```python
from build123d import *

# Parameters (mm, degrees)
SKETCH1_R                = 1.75
BOSS_EXTRUDE1_DEPTH      = 1.5
BOSS_EXTRUDE2_DEPTH      = 72
BOSS_EXTRUDE3_DEPTH      = 1.5
BOSS_EXTRUDE3_DEPTH_BACK = 1.5
BOSS_EXTRUDE4_DEPTH      = 2
SKETCH5_R                = 1.75
CUT_EXTRUDE1_DEPTH       = 2
CUT_EXTRUDE2_DEPTH       = 148.332054879
CUT_EXTRUDE2_DEPTH_BACK  = 148.332054879
SKETCH6_W                = 72
SKETCH6_H                = 11.553195909
BOSS_EXTRUDE6_START      = -2
SKETCH7_W                = 3
SKETCH7_H                = 4
BOSS_EXTRUDE6_DEPTH      = 2.5
FILLET1_R                = 2
CHAMFER1_SIZE            = 1
FILLET2_R                = 8
SKETCH8_W                = 35
SKETCH8_H                = 19.946804091
CUT_EXTRUDE3_DEPTH       = 22.4262221


with BuildPart() as part:
    # Sketch1 → Boss-Extrude1 (new body)
    with BuildSketch(Plane.XY):
        with BuildLine():
            Line((-31.5, -134.5), (31.5, -134.5))
            Line((31.5, -134.5), (36, -134.5))
            Line((36, -134.5), (36, -132.049019419))
            ThreePointArc((36, -132.049019419), (37.374296294, -129.5), (36, -126.950980581))
            Line((36, -126.950980581), (36, -6.049019419))
            ThreePointArc((36, -6.049019419), (37.33874188, -3.5), (36, -0.950980581))
            Line((36, -0.950980581), (36, 0))
            Line((36, 0), (-36, 0))
            Line((-36, 0), (-36, -0.950980581))
            ThreePointArc((-36, -0.950980581), (-37.339851511, -3.504206195), (-35.994020506, -6.054285021))
            Line((-35.994020506, -6.054285021), (-36, -126.950980581))
            ThreePointArc((-36, -126.950980581), (-37.376731289, -129.5), (-36, -132.049019419))
            Line((-36, -132.049019419), (-36, -134.5))
            Line((-36, -134.5), (-31.5, -134.5))
        make_face()
        with Locations((-34.328609587, -129.5)):
            Circle(SKETCH1_R, mode=Mode.SUBTRACT)
        with Locations((34.323211043, -129.5)):
            Circle(SKETCH1_R, mode=Mode.SUBTRACT)
        with Locations((34.242652207, -3.5)):
            Circle(SKETCH1_R, mode=Mode.SUBTRACT)
        with Locations((-34.244120111, -3.500578956)):
            Circle(SKETCH1_R, mode=Mode.SUBTRACT)
    extrude(amount=BOSS_EXTRUDE1_DEPTH)

    # Sketch2 → Boss-Extrude2 (add)
    with BuildSketch(Plane.ZY.offset(36)):
        Polygon((1.5, -134.5), (1.5, -136.7), (-40, -136.7), (-40, -134.7), (0, -134.7), (0, -134.5), (0, -132.049019419), (1.5, -132.049019419), align=None)
    extrude(amount=-BOSS_EXTRUDE2_DEPTH)

    # Sketch3 → Boss-Extrude3 (add, two sides: drawn at the far end of the back side and taken through both)
    with BuildSketch(Plane(origin=(0, 0, 0), x_dir=(0, 0, -1), z_dir=(1, 0, 0)).offset(-BOSS_EXTRUDE3_DEPTH_BACK)):
        Polygon((0, -119.7), (15, -134.7), (0, -134.7), align=None)
    extrude(amount=BOSS_EXTRUDE3_DEPTH + BOSS_EXTRUDE3_DEPTH_BACK)

    # Sketch4 → Boss-Extrude4 (add)
    with BuildSketch(Plane.XZ.offset(136.7)):
        with BuildLine():
            Line((-36, -17.152805247), (-36, -22.963011674))
            ThreePointArc((-36, -22.963011674), (-37.650416645, -20.05790846), (-36, -17.152805247))
        make_face()
        with BuildLine():
            Line((36, -17.152805247), (36, -22.963011674))
            ThreePointArc((36, -22.963011674), (37.68082264, -20.05790846), (36, -17.152805247))
        make_face()
    extrude(amount=-BOSS_EXTRUDE4_DEPTH)

    # Sketch5 → Cut-Extrude1 (cut)
    with BuildSketch(Plane.XZ.offset(136.7)):
        with Locations(Location((-34.253947115, -19.946804091, 0), (0, 0, 270))):
            Circle(SKETCH5_R)
        with Locations(Location((34.288977705, -19.889159472, 0), (0, 0, 270))):
            Circle(SKETCH5_R)
    extrude(amount=-CUT_EXTRUDE1_DEPTH, mode=Mode.SUBTRACT)

    # Sketch6 → Cut-Extrude2 (cut, two sides: drawn at the far end of the back side and taken through both)
    with BuildSketch(Plane.XZ.offset(136.7).offset(-CUT_EXTRUDE2_DEPTH_BACK)):
        with Locations((0, -34.223402046)):
            Rectangle(SKETCH6_W, SKETCH6_H)
    extrude(amount=CUT_EXTRUDE2_DEPTH + CUT_EXTRUDE2_DEPTH_BACK, mode=Mode.SUBTRACT)

    # Sketch7 → Boss-Extrude6 (add)
    with BuildSketch(Plane.XZ.offset(136.7).offset(BOSS_EXTRUDE6_START)):
        with Locations((-29.8, -26.446804091)):
            Rectangle(SKETCH7_W, SKETCH7_H)
        with Locations((29.8, -26.446804091)):
            Rectangle(SKETCH7_W, SKETCH7_H)
    extrude(amount=-BOSS_EXTRUDE6_DEPTH)

    # Fillet1
    fillet1_edges = [part.edges().sort_by_distance(p)[0] for p in [
        (36, -135.7, -28.446804091),
        (-36, -135.7, -28.446804091),
    ]]
    fillet(fillet1_edges, radius=FILLET1_R)

    # Chamfer1
    chamfer1_edges = [part.edges().sort_by_distance(p)[0] for p in [
        (-29.8, -134.7, -24.446804091),
        (-29.8, -132.2, -24.446804091),
        (29.8, -134.7, -24.446804091),
        (29.8, -132.2, -24.446804091),
    ]]
    chamfer(chamfer1_edges, length=CHAMFER1_SIZE)

    # Fillet2
    # the kernel refuses this fillet: 8 mm, written as the material it takes off along each edge
    with BuildSketch(Plane(origin=(-23.303909917, -133.2, -24.446804091), x_dir=(0, -1.0, -1.118394266079786e-11), z_dir=(-1, 0, 0))) as fillet2_piece_1:
        with BuildLine():
            CenterArc((4.243746579, -7.06996192), FILLET2_R, 117.902496562, 17.097503438)
            Line((-1.413107671, -1.413107671), (0, 0))
            Line((0, 0), (0.5, 0))
        make_face()
    extrude(amount=12.992180166, mode=Mode.SUBTRACT)
    with BuildSketch(Plane(origin=(23.303909917, -133.2, -24.446804091), x_dir=(0, 0.7071067811865476, -0.7071067811865476), z_dir=(1, 0, 0))) as fillet2_piece_2:
        with BuildLine():
            CenterArc((1.998436033, -8), FILLET2_R, 90, 17.097503438)
            Line((-0.353553391, -0.353553391), (0, 0))
            Line((0, 0), (1.998436033, 0))
        make_face()
    extrude(amount=12.992180166, mode=Mode.SUBTRACT)

    # Sketch8 → Cut-Extrude3 (cut)
    with BuildSketch(Plane.XZ.offset(136.7)):
        with Locations((-13.5, -15.473402046)):
            Rectangle(SKETCH8_W, SKETCH8_H)
    extrude(amount=-CUT_EXTRUDE3_DEPTH, mode=Mode.SUBTRACT)


solid = part.part
```
Could you check a few things on this model? Use its own coordinates, in mm. A direction names the side the tool comes from. Coordinates: 2 decimals unless noted, no trailing zeros. Write each loop counter-clockwise with the first axis right and the second up, starting at its lowest first coordinate (ties: lowest second). Pieces come first, ordered by that corner, then holes. Notation, with made-up numbers: (13.5, 31.25) -> (52.5, 31.25) arc R24 ccw to (52.5, 43.25) -> close; hole circle Ø3 at (-16, -16.75). An arc over 180 degrees is marked (long way). Return JSON: item names as keys, results as strings.
(1) I'm going to push flat-ended pins straight in: pin 1 (1.5 mm diameter, centred on x = -17, y = -24.5, fed in from -Z); pin 2 (2 mm diameter, centred on x = 34.24, y = -3.5, fed in from +Z); pin 3 (3.5 mm diameter, centred on y = -135, z = -3, fed in from +X); pin 4 (4.5 mm diameter, centred on y = -127, z = -2.5, fed in from -X). Where does each tip first touch, or does it pass through?
Numbers:
{"pin 1": "stops at z = 0", "pin 2": "passes through", "pin 3": "stops at x = 36", "pin 4": "stops at x = -1.5"}
(2) Imagine slicing it at D-D, the plane z = -2.5. Please give me the cut outline in (x, y).
Numbers:
{"outline": "(-36, -136.7) -> (36, -136.7) -> (36, -134.7) -> (1.5, -134.7) -> (1.5, -122.2) -> (-1.5, -122.2) -> (-1.5, -134.7) -> (-36, -134.7) -> close"}
(3) I need wall thicknesses on L1, parallel to X at y = -129.5, z = 1; L2, parallel to Y at x = -9, z = -2.5; L3, parallel to Z at x = -8, y = -128. Which ranges of each line are inside material? Lowest first, please.
Numbers:
{"L1": "x = -37.38 to -36.08, -32.58 to 32.57, 36.07 to 37.37", "L2": "y = -136.7 to -134.7", "L3": "z = 0 to 1.5"}
(4) Imagine slicing it at A-A, the plane y = -129.5. Please give me the cut outline in (x, z), then the cut area to 3 significant figures.
Numbers:
{"outline": "(-37.38, 0) -> (-36.08, 0) -> (-36.08, 1.5) -> (-37.38, 1.5) -> close; (-32.58, 0) -> (-1.5, 0) -> (-1.5, -5.5) -> (1.5, -5.5) -> (1.5, 0) -> (32.57, 0) -> (32.57, 1.5) -> (-32.58, 1.5) -> close; (36.07, 0) -> (37.37, 0) -> (37.37, 1.5) -> (36.07, 1.5) -> close", "area": "118 mm2"}
(5) Imagine slicing it at B-B, the plane x = -20.5. Please give me the cut outline in (y, z).
Numbers:
{"outline": "(-136.7, -28.45) -> (-134.7, -28.45) -> (-134.7, -25.45) -> (-136.7, -25.45) -> close; (-136.7, -5.5) -> (-134.7, -5.5) -> (-134.7, 0) -> (0, 0) -> (0, 1.5) -> (-136.7, 1.5) -> close"}
(6) We'd pull the mould along Y, two halves only. Please class faces 6 (the cylindrical face through (-33.52, -131.05, 0.74)), 7 (the cylindrical face through (-32.628, -4.171, 0.74)), 8 (the flat face through (-1, -66, 0)), 9 (the flat face through (30, -132.2, -27)): +Y half, -Y half, draft (parallel to the pull), parting line (faces both ways), or undercut.
Numbers:
{"face 6": "undercut", "face 7": "undercut", "face 8": "draft", "face 9": "+Y half"}
(7) Which directions (+Z, -Z, +X, -X, +Y, -Y) give clear straight access to the entire face, cutting with the end or side of a thin tool? Please do faces 1 (the flat face through (-28.3, -133, -27)), 2 (the flat face through (31.3, -133, -27)), 3 (the flat face through (36, -135, -8)), 4 (the flat face through (-31.3, -133, -27)), 5 (the flat face through (-14, -135, -25.447)).
Numbers:
{"face 1": "-Z, +Y", "face 2": "-Z, +X, +Y", "face 3": "+Z, +X, -Y", "face 4": "-Z, -X, +Y", "face 5": "+Y, -Y"}
(8) Imagine slicing it at C-C, the plane z = -9.25. Please give me the cut outline in (x, y), then the cut area to 3 significant figures.
Numbers:
{"outline": "(-36, -136.7) -> (-31, -136.7) -> (-31, -134.7) -> (-36, -134.7) -> close; (4, -136.7) -> (36, -136.7) -> (36, -134.7) -> (4, -134.7) -> close", "area": "74.0 mm2"}
